Read the model definition and answer for the solid it produces. Units are mm, in the model's axes. A direction names the side the tool comes from. Give positions to 0.01 mm unless a question says otherwise; leave off trailing zeros. Order: outer loops, then holes, each group sorted by start corner. A loop starts at its lowest first (then second) coordinate and runs counter-clockwise, first axis right, second up.
```python
from build123d import *

# Parameters (mm, degrees)
BOSS_EXTRUDE1_DEPTH = 279.4
CUT_EXTRUDE1_REACH  = 78.2
SKETCH2_R           = 9.525
CUT_EXTRUDE2_REACH  = 154.4
SKETCH3_R           = 9.525


with BuildPart() as part:
    # Sketch1 → Boss-Extrude1 (new body, symmetric)
    with BuildSketch(Plane(origin=(0, 0, 0), x_dir=(0, 0, -1), z_dir=(1, 0, 0))):
        with BuildLine():
            Line((-48.8061, -76.2), (-48.8061, 76.2))
            Line((-48.8061, 76.2), (27.3939, 76.2))
            Line((27.3939, 76.2), (27.3939, 73.710744653))
            ThreePointArc((27.3939, 73.710744653), (26.61173954, 71.672050174), (24.666685315, 70.679672107))
            Line((24.666685315, 70.679672107), (-29.288063286, 64.969518115))
            ThreePointArc((-29.288063286, 64.969518115), (-34.150698849, 62.488572947), (-36.1061, 57.391836749))
            Line((-36.1061, 57.391836749), (-36.1061, -57.391836749))
            ThreePointArc((-36.1061, -57.391836749), (-34.150698849, -62.488572947), (-29.288063286, -64.969518115))
            Line((-29.288063286, -64.969518115), (24.666685315, -70.679672107))
            ThreePointArc((24.666685315, -70.679672107), (26.61173954, -71.672050174), (27.3939, -73.710744653))
            Line((27.3939, -73.710744653), (27.3939, -76.2))
            Line((27.3939, -76.2), (-48.8061, -76.2))
        make_face()
    extrude(amount=BOSS_EXTRUDE1_DEPTH, both=True)

    # Sketch2 → Cut-Extrude1 (cut, up to next)
    with BuildSketch(Plane.XY.offset(48.8061), mode=Mode.PRIVATE) as cut_extrude1_sk1:
        with Locations((-254, 30.1625)):
            Circle(SKETCH2_R)
    cut_extrude1_tool1 = extrude(cut_extrude1_sk1.sketch, amount=-CUT_EXTRUDE1_REACH, mode=Mode.PRIVATE) & part.part
    add(cut_extrude1_tool1.solids().sort_by_distance((-254, 30.1625, 48.8061))[0], mode=Mode.SUBTRACT)
    # Sketch2 → Cut-Extrude1 (cut, up to next)
    with BuildSketch(Plane.XY.offset(48.8061), mode=Mode.PRIVATE) as cut_extrude1_sk2:
        with Locations((-254, -30.1625)):
            Circle(SKETCH2_R)
    cut_extrude1_tool2 = extrude(cut_extrude1_sk2.sketch, amount=-CUT_EXTRUDE1_REACH, mode=Mode.PRIVATE) & part.part
    add(cut_extrude1_tool2.solids().sort_by_distance((-254, -30.1625, 48.8061))[0], mode=Mode.SUBTRACT)
    # Sketch2 → Cut-Extrude1 (cut, up to next)
    with BuildSketch(Plane.XY.offset(48.8061), mode=Mode.PRIVATE) as cut_extrude1_sk3:
        with Locations((254, -30.1625)):
            Circle(SKETCH2_R)
    cut_extrude1_tool3 = extrude(cut_extrude1_sk3.sketch, amount=-CUT_EXTRUDE1_REACH, mode=Mode.PRIVATE) & part.part
    add(cut_extrude1_tool3.solids().sort_by_distance((254, -30.1625, 48.8061))[0], mode=Mode.SUBTRACT)
    # Sketch2 → Cut-Extrude1 (cut, up to next)
    with BuildSketch(Plane.XY.offset(48.8061), mode=Mode.PRIVATE) as cut_extrude1_sk4:
        with Locations((254, 30.1625)):
            Circle(SKETCH2_R)
    cut_extrude1_tool4 = extrude(cut_extrude1_sk4.sketch, amount=-CUT_EXTRUDE1_REACH, mode=Mode.PRIVATE) & part.part
    add(cut_extrude1_tool4.solids().sort_by_distance((254, 30.1625, 48.8061))[0], mode=Mode.SUBTRACT)

    # Sketch3 → Cut-Extrude2 (cut, up to next)
    with BuildSketch(Plane.XZ.offset(76.2), mode=Mode.PRIVATE) as cut_extrude2_sk1:
        with Locations((-165.1, 10.7061)):
            Circle(SKETCH3_R)
    cut_extrude2_tool1 = extrude(cut_extrude2_sk1.sketch, amount=-CUT_EXTRUDE2_REACH, mode=Mode.PRIVATE) & part.part
    add(cut_extrude2_tool1.solids().sort_by_distance((-165.1, -76.2, 10.7061))[0], mode=Mode.SUBTRACT)
    # Sketch3 → Cut-Extrude2 (cut, up to next)
    with BuildSketch(Plane.XZ.offset(76.2), mode=Mode.PRIVATE) as cut_extrude2_sk2:
        with Locations((165.1, 10.7061)):
            Circle(SKETCH3_R)
    cut_extrude2_tool2 = extrude(cut_extrude2_sk2.sketch, amount=-CUT_EXTRUDE2_REACH, mode=Mode.PRIVATE) & part.part
    add(cut_extrude2_tool2.solids().sort_by_distance((165.1, -76.2, 10.7061))[0], mode=Mode.SUBTRACT)


solid = part.part
```
1) The part is cut by section D-D on y = -50. Determine the outline of the cut face in (x, z).
Final values:
outline: (-279.4, 36.11) - (279.4, 36.11) - (279.4, 48.81) - (-279.4, 48.81) - close
2) Given pin 1 (10 mm diameter, centred on x = 47.5, y = -38.5, fed in from -Z); pin 2 (25 mm diameter, centred on x = 254, y = 30.16, fed in from +Z); pin 3 (15 mm diameter, centred on x = 165.1, z = 10.71, fed in from -Y), each flat-ended and moving along its own axis, determine where each tip first touches the part or whether it passes through.
Final values:
pin 1: stops at z = 36.11
pin 2: stops at z = 48.81
pin 3: stops at y = 66.14
3) The part is cut by section C-C on x = 160.5. Determine the outline of the cut face in (y, z).
Final values:
outline: (-76.2, -27.39) - (-73.71, -27.39) arc R3.05 ccw to (-70.68, -24.67) - (-67.82, 2.37) - (-76.2, 2.37) - close; (-76.2, 19.05) - (-66.05, 19.05) - (-64.97, 29.29) arc R7.62 cw to (-57.39, 36.11) - (57.39, 36.11) arc R7.62 cw to (64.97, 29.29) - (70.68, -24.67) arc R3.05 ccw to (73.71, -27.39) - (76.2, -27.39) - (76.2, 48.81) - (-76.2, 48.81) - close
4) Consider L1, parallel to Y at x = -254, z = 41; L2, parallel to Z at x = 67, y = 19.5; L3, parallel to Y at x = -6.5, z = 13. Determine where each line is inside the solid, lowest interval first.
Final values:
L1: y = -76.2 to -39.69, -20.64 to 20.64, 39.69 to 76.2
L2: z = 36.11 to 48.81
L3: y = -76.2 to -66.69, 66.69 to 76.2
5) A tool of negligible diameter and unlimited length cuts with its end or side. For faces 4 (the face through (279.4, -5, 39)), 5 (the face through (163.86, -71.14, 20.15)), 6 (the face through (3.912, -67.785, 2.688)), from which of +Z, -Z, +X, -X, +Y, -Y can it reach the whole face along a straight path? Write none if from no direction.
Final values:
face 4: +Z, -Z, +X, +Y, -Y
face 5: -Y
face 6: -Z, +X, -X
6) For a pull along Z with two mould halves and no side action, classify faces 1 (the face through (246.98, 36.6, 42.54)), 2 (the face through (3.912, 67.865, 1.933)), 3 (the face through (-166.34, -71.14, 20.15)) as released by +Z, released by -Z, zero draft, split by the parting line, or undercut.
Final values:
face 1: zero draft
face 2: released by -Z
face 3: undercut
7) The part is cut by section B-B on x = -37. Determine the outline of the cut face in (y, z).
Final values:
outline: (-76.2, -27.39) - (-73.71, -27.39) arc R3.05 ccw to (-70.68, -24.67) - (-64.97, 29.29) arc R7.62 cw to (-57.39, 36.11) - (57.39, 36.11) arc R7.62 cw to (64.97, 29.29) - (70.68, -24.67) arc R3.05 ccw to (73.71, -27.39) - (76.2, -27.39) - (76.2, 48.81) - (-76.2, 48.81) - close
8) The part is cut by section A-A on x = 254. Determine the outline of the cut face in (y, z), and give its area (3 significant figures).
Final values:
outline: (-76.2, -27.39) - (-73.71, -27.39) arc R3.05 ccw to (-70.68, -24.67) - (-64.97, 29.29) arc R7.62 cw to (-57.39, 36.11) - (-39.69, 36.11) - (-39.69, 48.81) - (-76.2, 48.81) - close; (-20.64, 36.11) - (20.64, 36.11) - (20.64, 48.81) - (-20.64, 48.81) - close; (39.69, 36.11) - (57.39, 36.11) arc R7.62 cw to (64.97, 29.29) - (70.68, -24.67) arc R3.05 ccw to (73.71, -27.39) - (76.2, -27.39) - (76.2, 48.81) - (39.69, 48.81) - close
area: 2,560 mm2
